Part model, mm, in its own coordinate system. Face numbers are marked on the shaded views. Give positions to 0.01 mm unless a question says otherwise; leave off trailing zeros. Write each loop counter-clockwise with the first axis right and the second up, starting at its lowest first coordinate (ties: lowest second). Pieces come first, ordered by that corner, then holes. Notation, with made-up numbers: M -31,-38.75 L 20,-38.75 A28 ccw 20,-17.75 Z; hole C 71,-6.5 d1. An arc over 180 degrees is marked long. Write item = value, one per line. Start each with the question number.
from build123d import *

# Parameters (mm, degrees)
F0_R     = 4.6
F1_DEPTH = 12.7
F0_R_2   = 3.2
F2_DEPTH = 1


with BuildPart() as f1:
    # F0 (on Top) → F1 (new body)
    with BuildSketch(Plane.XY):
        Polygon((3.4063665882, 5.9), (-3.4063665882, 5.9), (-6.8127331764, 0), (-3.4063665882, -5.9), (3.4063665882, -5.9), (6.8127331764, 0), align=None)
        Circle(F0_R, mode=Mode.SUBTRACT)
    extrude(amount=F1_DEPTH)

    # F0 (on Top) → F2 (join)
    with BuildSketch(Plane.XY):
        Polygon((3.4063665882, 5.9), (-3.4063665882, 5.9), (-6.8127331764, 0), (-3.4063665882, -5.9), (3.4063665882, -5.9), (6.8127331764, 0), align=None)
        Circle(F0_R, mode=Mode.SUBTRACT)
        Circle(F0_R)
        Circle(F0_R_2, mode=Mode.SUBTRACT)
    extrude(amount=-F2_DEPTH)


solid = f1.part
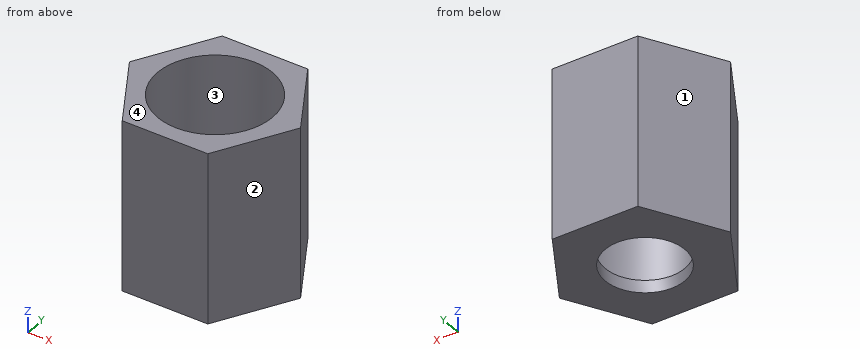
Q1. Slice it at D-D (x = -5). Give the cut face in (y, z), and give its area (3 significant figures).
Q2. Slice it at A-A (x = 0). Give the cut face in (y, z), and give its area (3 significant figures).
Q3. Probe line 1 along Y through (x, z) = (0, -0.25); line 2 along Y through (x, z) = (0, 9.75); line 3 along X through (y, z) = (-2.25, 7). List the from-to ranges inside material, lowest first.
Q4. Two-plate mould, pull along X, no slides. Class the marked faces 1, 2, 3 and 4: +X half, -X half, draft (parallel to the pull), parting line (faces both ways), or undercut.
Q5. Drop flat-ended pins along their axis: P1, Ø3, axis at x = 2, y = 0, coming from the +Z side; P2, Ø2, axis at y = -1.5, z = 8, coming from the -X side; P3, Ø1.5, axis at y = 2.5, z = 1, coming from the +X side. Give the stop position or say it passes through.
Q6. Slice it at B-B (z = 11.75). Give the cut face in (x, y), and give its area (3 significant figures).
Q7. Slice it at C-C (y = -2.5). Give the cut face in (x, z).
Working result:
q1.outline = M -3.14,-1 L 3.14,-1 L 3.14,12.7 L -3.14,12.7 Z
q1.area = 86.0 mm2
q2.outline = M -5.9,-1 L -3.2,-1 L -3.2,0 L -4.6,0 L -4.6,12.7 L -5.9,12.7 Z; M 3.2,-1 L 5.9,-1 L 5.9,12.7 L 4.6,12.7 L 4.6,0 L 3.2,0 Z
q2.area = 38.4 mm2
q3.line_1 = -5.9 to -3.2, 3.2 to 5.9
q3.line_2 = -5.9 to -4.6, 4.6 to 5.9
q3.line_3 = -5.51 to -4.01, 4.01 to 5.51
q4.face_1 = -X half
q4.face_2 = +X half
q4.face_3 = undercut
q4.face_4 = draft
q5.P1 = 0
q5.P2 = -6.52
q5.P3 = 5.8
q6.outline = M -6.81,0 L -3.41,-5.9 L 3.41,-5.9 L 6.81,0 L 3.41,5.9 L -3.41,5.9 Z; hole C 0,0 d9.2
q6.area = 54.1 mm2
q7.outline = M -5.37,-1 L -2,-1 L -2,0 L -3.86,0 L -3.86,12.7 L -5.37,12.7 Z; M 2,-1 L 5.37,-1 L 5.37,12.7 L 3.86,12.7 L 3.86,0 L 2,0 Z
